Could you check a few things on this model? Use its own coordinates, in mm. Face numbers are marked on the shaded views. A direction names the side the tool comes from. Give positions to 0.01 mm unless a question says otherwise; leave off trailing zeros. Order: outer loops, then holes, each group sorted by start corner. A loop starts at its lowest first (then second) coordinate and runs counter-clockwise, first axis right, second up. Notation, with made-up numbers: M -14,20.5 L 26,20.5 A10 cw 26,30.5 Z; hole C 42.25,-11 d6. An arc over 180 degrees is marked long. Use a Markdown table: item, result. Add a question column.
Item 1: For the marked faces 5, 6, 7, 8 and 9, which set-ups out of +Z, -Z, +X, -X, +Y, -Y let a thin tool reach every point of the face, with its end or its side?
Item 2: Suppose I cut it at C-C on y = 7.5. Write out the boundary of the cut face in (x, z), plus the area to 3 significant figures.
Item 3: Suppose I cut it at A-A on z = 0. Write out the boundary of the cut face in (x, y).
Item 4: Suppose I cut it at B-B on x = 0. Write out the boundary of the cut face in (y, z), plus the area to 3 significant figures.
Item 5: If I drill on L1, parallel to X at y = 24, z = 0; L2, parallel to X at y = 26.5, z = 22, over which ranges is the centre line in solid material (lowest first)? Write a range as from..to.
Item 6: Suppose I cut it at D-D on x = 6. Write out the boundary of the cut face in (y, z).
Item 7: If we mould it in two halves opening along Z, with no side actions, what happens to the marked faces 1, 2, 3 and 4? For each: released by +Z, released by -Z, zero draft, split by the parting line, or undercut.
Item 8: I'm going to push flat-ended pins straight in: pin 1 Ø3 at (x, z) = (-20.5, 1.5) entering from +Y; pin 2 Ø10 at (y, z) = (36, -21.5) entering from +X; pin 3 Ø2 at (x, y) = (2, 8.5) entering from +Z; pin 4 Ø7 at (x, z) = (0, 0) entering from -Y. Where does each tip first touch, or does it pass through?
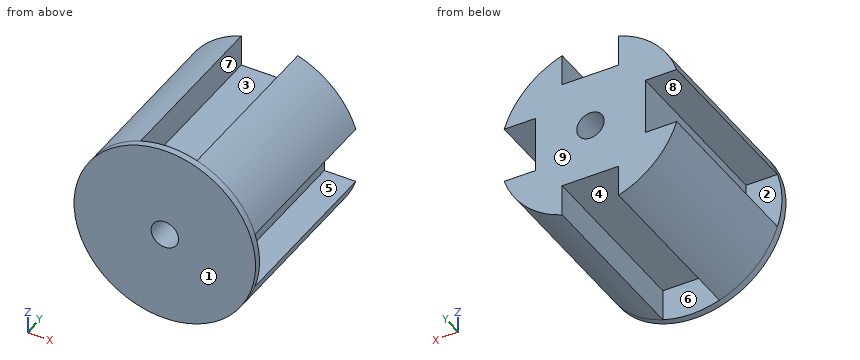
from build123d import *

# Parameters (mm, degrees)
BOSS_EXTRUDE1_DEPTH = 51
SKETCH3_R           = 26.5
BOSS_EXTRUDE2_DEPTH = 2
SKETCH4_R           = 4
CUT_EXTRUDE1_DEPTH  = 54


with BuildPart() as part:
    # Sketch2 → Boss-Extrude1 (new body)
    with BuildSketch(Plane(origin=(0, 0, 0), x_dir=(1, 0, 0), z_dir=(0, 1, 0))):
        with BuildLine():
            Line((-8.25, 25.183079637), (-8.25, 16))
            Line((-8.25, 16), (8.25, 16))
            Line((8.25, 16), (8.25, 25.183079637))
            ThreePointArc((8.25, 25.183079637), (18.738329701, 18.738329701), (25.183079637, 8.25))
            Line((25.183079637, 8.25), (16, 8.25))
            Line((16, 8.25), (16, -8.25))
            Line((16, -8.25), (25.183079637, -8.25))
            ThreePointArc((25.183079637, -8.25), (18.738329701, -18.738329701), (8.25, -25.183079637))
            Line((8.25, -25.183079637), (8.25, -16))
            Line((8.25, -16), (-8.25, -16))
            Line((-8.25, -16), (-8.25, -25.183079637))
            ThreePointArc((-8.25, -25.183079637), (-18.738329701, -18.738329701), (-25.183079637, -8.25))
            Line((-25.183079637, -8.25), (-16, -8.25))
            Line((-16, -8.25), (-16, 8.25))
            Line((-16, 8.25), (-25.183079637, 8.25))
            ThreePointArc((-25.183079637, 8.25), (-18.738329701, 18.738329701), (-8.25, 25.183079637))
        make_face()
    extrude(amount=BOSS_EXTRUDE1_DEPTH)

    # Sketch3 → Boss-Extrude2 (add)
    with BuildSketch(Plane.XZ):
        Circle(SKETCH3_R)
    extrude(amount=BOSS_EXTRUDE2_DEPTH)

    # Sketch4 → Cut-Extrude1 (cut, through all)
    with BuildSketch(Plane(origin=(0, 51, 0), x_dir=(1, 0, 0), z_dir=(0, 1, 0))):
        Circle(SKETCH4_R)
    extrude(amount=-CUT_EXTRUDE1_DEPTH, mode=Mode.SUBTRACT)


solid = part.part
Findings below:
| question | item | result |
|---|---|---|
| 1 | face 5 | +X, +Y |
| 1 | face 6 | -Z, +Y |
| 1 | face 7 | +Z, +Y |
| 1 | face 8 | -X, +Y |
| 1 | face 9 | +Z, -Z, +X, -X, +Y |
| 2 | outline | M -25.18,-8.25 A26.5 ccw -8.25,-25.18 L -8.25,-16 L 8.25,-16 L 8.25,-25.18 A26.5 ccw 25.18,-8.25 L 16,-8.25 L 16,8.25 L 25.18,8.25 A26.5 ccw 8.25,25.18 L 8.25,16 L -8.25,16 L -8.25,25.18 A26.5 ccw -25.18,8.25 L -16,8.25 L -16,-8.25 Z; hole C 0,0 d8 |
| 2 | area | 1,490 mm^2 |
| 3 | outline | M -26.5,-2 L -4,-2 L -4,51 L -16,51 L -16,0 L -26.5,0 Z; M 4,-2 L 26.5,-2 L 26.5,0 L 16,0 L 16,51 L 4,51 Z |
| 4 | outline | M -2,-26.5 L 0,-26.5 L 0,-16 L 51,-16 L 51,-4 L -2,-4 Z; M -2,4 L 51,4 L 51,16 L 0,16 L 0,26.5 L -2,26.5 Z |
| 4 | area | 1,310 mm^2 |
| 5 | L1 | x = -16..-4, 4..16 |
| 5 | L2 | x = -14.77..-8.25, 8.25..14.77 |
| 6 | outline | M -2,-25.81 L 0,-25.81 L 0,-16 L 51,-16 L 51,16 L 0,16 L 0,25.81 L -2,25.81 Z |
| 7 | face 1 | zero draft |
| 7 | face 2 | undercut |
| 7 | face 3 | released by +Z |
| 7 | face 4 | released by -Z |
| 8 | pin 1 | stops at y = 0 |
| 8 | pin 2 | stops at x = 20.74 |
| 8 | pin 3 | stops at z = 16 |
| 8 | pin 4 | passes through |
